Could you check a few things on this drawing? It's one solid part, dimensions in mm from its lowest x, y, z. A direction names the side the tool comes from. Round coordinates to 2 decimals unless told otherwise and drop trailing zeros. Write each loop counter-clockwise with the first axis right and the second up, starting at its lowest first coordinate (ties: lowest second). Pieces come first, ordered by that corner, then holes. Notation, with made-up numbers: (-26, 38) -> (-16, 38) arc R25 cw to (-16, 52) -> close; hole circle Ø9 at (-34.75, 24). An arc over 180 degrees is marked (long way). Put each result on its own line as item: value. Start each with the question number.
1) If I drill on line 1 along Z through (x, y) = (8.5, 13.65); line 2 along Z through (x, y) = (14.5, 7.25); line 3 along X through (y, z) = (10.75, 1.5), over which ranges is the centre line in solid material (lowest first)? Write a range as [from, to].
2) I want a section at C-C, the plane z = 6.5. List the corners of the cut face in (x, y) for me.
3) Will these pins go through, and if not, where does the flat tip stop? P1, Ø2, axis at y = 8.5, z = 6.5, coming from the +X side; P2, Ø2, axis at x = 14, z = 6, coming from the +Y side; P3, Ø1.5, axis at x = 8.5, z = 6.5, coming from the -Y side.
4) We'd pull the mould along X, two halves only. Please class the marked faces 1, 2, 3 and 4: released by +X, released by -X, zero draft, split by the parting line, or undercut.
5) I want a section at A-A, the plane y = 8.5. List the corners of the cut face in (x, z) for me, then the cut area to 3 significant figures.
6) I want a section at D-D, the plane x = 4.75. List the corners of the cut face in (y, z) for me, then the cut area to 3 significant figures.
7) Which directions (+Z, -Z, +X, -X, +Y, -Y) give clear straight access to the entire face, cutting with the end or side of a thin tool? Please do the marked faces 5 and 6.
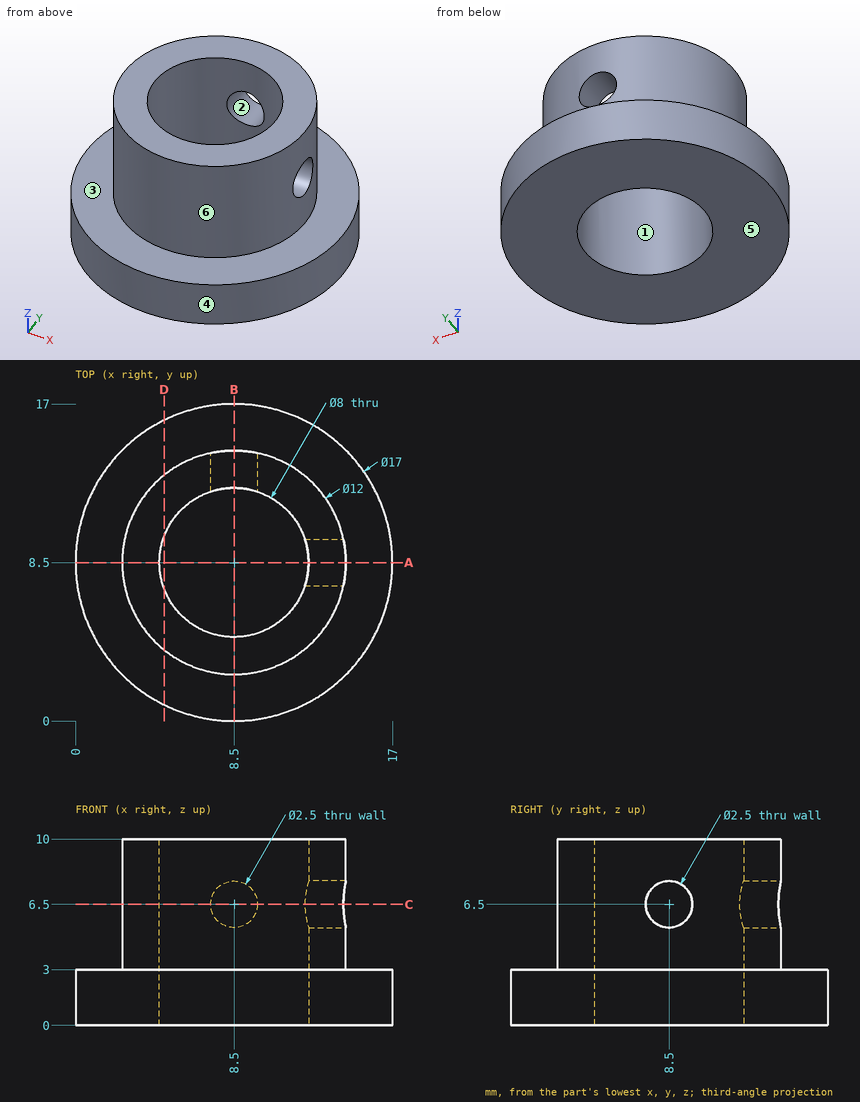
Findings:
1. line 1: z = [0, 5.25], [7.75, 10]
1. line 2: z = [0, 3]
1. line 3: x = [0.3, 5.19], [11.81, 16.7]
2. outline: (7.25, 12.3) -> (7.25, 14.37) arc R6 ccw (long way) to (14.37, 7.25) -> (12.3, 7.25) arc R4 cw (long way) to start; (9.75, 12.3) arc R4 cw to (12.3, 9.75) -> (14.37, 9.75) arc R6 ccw to (9.75, 14.37) -> close
3. P1: stops at x = 4.63
3. P2: stops at y = 12.47
3. P3: stops at y = 2.5
4. face 1: undercut
4. face 2: undercut
4. face 3: zero draft
4. face 4: split by the parting line
5. outline: (0, 0) -> (4.5, 0) -> (4.5, 10) -> (2.5, 10) -> (2.5, 3) -> (0, 3) -> close; (12.5, 0) -> (17, 0) -> (17, 3) -> (14.5, 3) -> (14.5, 5.25) -> (12.5, 5.25) -> close; (12.5, 7.75) -> (14.5, 7.75) -> (14.5, 10) -> (12.5, 10) -> close
5. area: 50.0 mm2
6. outline: (0.87, 0) -> (7.11, 0) -> (7.11, 10) -> (3.82, 10) -> (3.82, 3) -> (0.87, 3) -> close; (9.89, 0) -> (16.13, 0) -> (16.13, 3) -> (13.18, 3) -> (13.18, 10) -> (9.89, 10) -> close
6. area: 83.5 mm2
7. face 5: -Z, +X, -X, +Y, -Y
7. face 6: +Z
